from build123d import *

# Parameters (mm, degrees)
BOSS_EXTRUDE1_DEPTH     = 20
SKETCH3_R               = 20
CUT_EXTRUDE2_DEPTH      = 1
CUT_EXTRUDE2_DEPTH_BACK = 21
SKETCH4_R               = 12.5
CUT_EXTRUDE3_DEPTH      = 21


with BuildPart() as part:
    # Sketch1 → Boss-Extrude1 (new body)
    with BuildSketch(Plane.XY):
        with BuildLine():
            Line((35, -40), (-35, -40))
            ThreePointArc((-35, -40), (-45.606601718, -35.606601718), (-50, -25))
            Line((-50, -25), (-50, 25))
            ThreePointArc((-50, 25), (-45.606601718, 35.606601718), (-35, 40))
            Line((-35, 40), (35, 40))
            ThreePointArc((35, 40), (45.606601718, 35.606601718), (50, 25))
            Line((50, 25), (50, -25))
            ThreePointArc((50, -25), (45.606601718, -35.606601718), (35, -40))
        make_face()
    extrude(amount=BOSS_EXTRUDE1_DEPTH)

    # Sketch3 → Cut-Extrude2 (cut, two sides)
    with BuildSketch(Plane.XY.offset(20)) as cut_extrude2_sk:
        with Locations((-10, 0)):
            Circle(SKETCH3_R)
    extrude(amount=CUT_EXTRUDE2_DEPTH, mode=Mode.SUBTRACT)
    extrude(cut_extrude2_sk.sketch, amount=-CUT_EXTRUDE2_DEPTH_BACK, mode=Mode.SUBTRACT)

    # Sketch4 → Cut-Extrude3 (cut, through all)
    with BuildSketch(Plane.XY.offset(20)):
        with Locations((30, 0)):
            Circle(SKETCH4_R)
    extrude(amount=-CUT_EXTRUDE3_DEPTH, mode=Mode.SUBTRACT)


solid = part.part
Design review of the part built by this model. Coordinates are the model's own, in mm. Give positions to 0.01 mm unless a question says otherwise; leave off trailing zeros. Loops run counter-clockwise (first coordinate to the right, second up) from the corner with the lowest first, then second, coordinate; pieces in that order, holes last. Notation, with made-up numbers: (14, 2) - (49, 2) arc R18 cw to (49, 15) - close; hole circle Ø11 at (80, -11). An arc over 180 degrees is marked (long way). Write item = value, one per line.
1) Take a section at C-C on z = 9. State the section outline as (x, y) points, and give its area (3 significant figures).
Result sheet:
outline = (-50, -25) arc R15 ccw to (-35, -40) - (35, -40) arc R15 ccw to (50, -25) - (50, 25) arc R15 ccw to (35, 40) - (-35, 40) arc R15 ccw to (-50, 25) - close; hole circle Ø40 at (-10, 0); hole circle Ø25 at (30, 0)
area = 6,060 mm2
2) Take a section at D-D on x = 30. State the section outline as (y, z) points.
Result sheet:
outline = (-40, 0) - (-12.5, 0) - (-12.5, 20) - (-40, 20) - close; (12.5, 0) - (40, 0) - (40, 20) - (12.5, 20) - close
3) Clearance check with a flat-ended pin moving along its axis: pin 1 Ø10 at (x, y) = (-22, -15.5) entering from +Z. State where the tip first meets the part, or that it passes through.
Result sheet:
pin_1 = 20
4) Draft analysis for pull direction X (two halves, no side actions). For faces 1 (the face through (20.08, -7.606, 10.14)), 2 (the face through (-50, 0, 10)), 3 (the face through (45.72, -35.49, 9.86)), state which applies: +X half, -X half, draft (parallel to the pull), parting line (faces both ways), or undercut.
Result sheet:
face_1 = undercut
face_2 = -X half
face_3 = +X half
5) To check wall thickness, follow line 1 (Y direction, x = -10, z = 10); line 2 (X direction, y = -15, z = 1); line 3 (X direction, y = 11, z = 9.75). State the ranges of each line that lie inside material, in increasing order.
Result sheet:
line_1 = -40 to -20, 20 to 40
line_2 = -50 to -23.23, 3.23 to 50
line_3 = -50 to -26.7, 6.7 to 24.06, 35.94 to 50
6) Take a section at B-B on y = 0. State the section outline as (x, z) points.
Result sheet:
outline = (-50, 0) - (-30, 0) - (-30, 20) - (-50, 20) - close; (10, 0) - (17.5, 0) - (17.5, 20) - (10, 20) - close; (42.5, 0) - (50, 0) - (50, 20) - (42.5, 20) - close
7) Take a section at A-A on x = -10. State the section outline as (y, z) points.
Result sheet:
outline = (-40, 0) - (-20, 0) - (-20, 20) - (-40, 20) - close; (20, 0) - (40, 0) - (40, 20) - (20, 20) - close
